Check sheet for the drawn part. Datum: minimum x, y, z corner. Units: mm. A direction names the side the tool comes from. Coordinates: 2 decimals unless noted, no trailing zeros. Write each loop counter-clockwise with the first axis right and the second up, starting at its lowest first coordinate (ties: lowest second). Pieces come first, ordered by that corner, then holes. Notation, with made-up numbers: M 88,54.25 L 135,54.25 A38 ccw 135,93.25 Z; hole C 60.25,32 d9. An arc over 180 degrees is marked long. Answer as CSV lines item,"result".
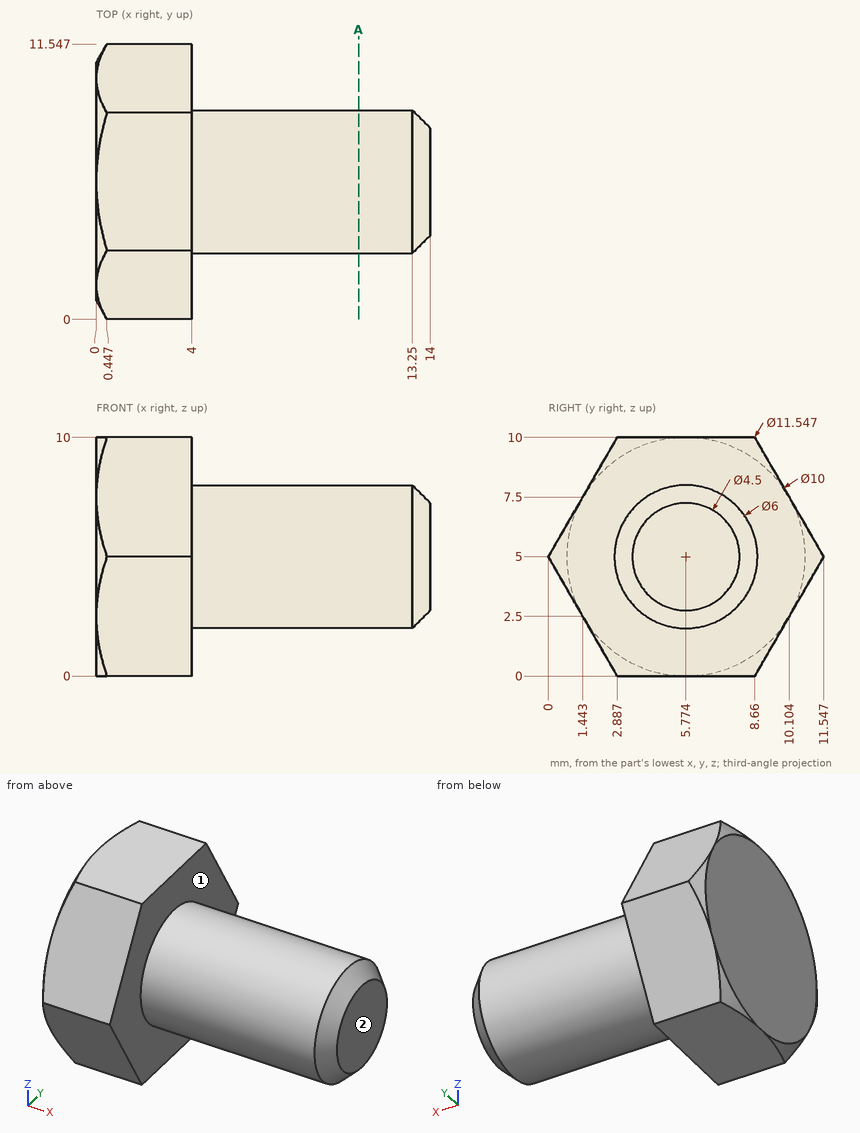
1) Thickness scan on line 1 along X through (y, z) = (7.25, 2.25); line 2 along Y through (x, z) = (2.5, 8) (1 decimal); line 3 along Y through (x, z) = (7, 4.75) (1 decimal). Record the ranges inside material, lowest first.
Answer key:
line 1,"x = 0 to 4"
line 2,"y = 1.7 to 9.8"
line 3,"y = 2.8 to 8.8"
2) Section check A-A, the plane x = 11. Record the boundary of the cut face in (y, z).
Answer key:
outline,"C 5.77,5 d6"
3) Tool access check on the marked faces 1 and 2. Record the directions out of +Z, -Z, +X, -X, +Y, -Y that give a thin tool (end or side, any length) a straight path to the whole face; none if there is none.
Answer key:
face 1,"+X"
face 2,"+Z, -Z, +X, +Y, -Y"
4) Depth check by flat-ended pin: P1, Ø4, axis at x = 10, z = 2, coming from the +Y side; P2, Ø1, axis at x = 8, y = 4, coming from the +Z side; P3, Ø4, axis at x = 8.5, y = 2.5, coming from the -Z side. Enter the tip coordinate at first touch or a pass-through.
Answer key:
P1,"stops at y = 8.6"
P2,"stops at z = 7.72"
P3,"stops at z = 2.28"
